```python
from build123d import *

# Parameters (mm, degrees)
SKETCH1_R           = 2.38125
SKETCH1_R_2         = 3.175
BOSS_EXTRUDE1_DEPTH = 3.175
FILLET1_R           = 7.62


with BuildPart() as part:
    # Sketch1 → Boss-Extrude1 (new body)
    with BuildSketch(Plane.XY):
        Polygon((0, 0), (25.4, 0), (25.4, -50.8), (50.8, -50.8), (50.8, -17.819677815), (65.055742252, 0), (65.055742252, 81.319677815), align=None)
        with Locations((15.875, 9.525)):
            Circle(SKETCH1_R, mode=Mode.SUBTRACT)
        with Locations((46.005742252, 38.1)):
            Circle(SKETCH1_R_2, mode=Mode.SUBTRACT)
        with Locations((46.005742252, 12.7)):
            Circle(SKETCH1_R_2, mode=Mode.SUBTRACT)
        with Locations((38.1, -12.7)):
            Circle(SKETCH1_R_2, mode=Mode.SUBTRACT)
        with Locations((38.1, -38.1)):
            Circle(SKETCH1_R_2, mode=Mode.SUBTRACT)
    extrude(amount=BOSS_EXTRUDE1_DEPTH)

    # Fillet1
    fillet1_edges = [part.edges().sort_by_distance(p)[0] for p in [
        (65.055742252, 81.319677815, 1.5875),
        (65.055742252, 0, 1.5875),
        (50.8, -17.819677815, 1.5875),
    ]]
    fillet(fillet1_edges, radius=FILLET1_R)


solid = part.part
```
Work out the finished part from the listing and answer in its coordinate system (mm). A direction names the side the tool comes from. Give positions to 0.01 mm unless a question says otherwise; leave off trailing zeros. Write each loop counter-clockwise with the first axis right and the second up, starting at its lowest first coordinate (ties: lowest second). Pieces come first, ordered by that corner, then holes.
(1) The part is cut by section D-D on y = -38.1. Write down the section's boundary in (x, z) (3 decimals), plus the area to 3 significant figures.
Final values:
outline: (25.4, 0) - (34.925, 0) - (34.925, 3.175) - (25.4, 3.175) - close; (41.275, 0) - (50.8, 0) - (50.8, 3.175) - (41.275, 3.175) - close
area: 60.5 mm2
(2) The part is cut by section B-B on x = 44. Write down the section's boundary in (y, z) (3 decimals), plus the area to 3 significant figures.
Final values:
outline: (-50.8, 0) - (10.239, 0) - (10.239, 3.175) - (-50.8, 3.175) - close; (15.161, 0) - (35.639, 0) - (35.639, 3.175) - (15.161, 3.175) - close; (40.561, 0) - (55, 0) - (55, 3.175) - (40.561, 3.175) - close
area: 305 mm2
(3) Flat-ended cylindrical pins translate along their axes: pin 1 Ø1.5 at (x, z) = (29, 1.5) entering from +Y; pin 2 Ø1.6 at (y, z) = (-23.5, 1.5) entering from -X; pin 3 Ø1 at (x, z) = (15.5, 1.5) entering from -Y. Find the tip coordinate at first contact, or state that the pin passes through.
Final values:
pin 1: stops at y = 37.19
pin 2: stops at x = 25.4
pin 3: stops at y = 0
(4) The part is cut by section C-C on z = 2. Count the separate pieces of the cut face and the enclosed holes in it, plus the area to 3 significant figures.
Final values:
separate pieces: 1
enclosed holes: 5
area: 3,820 mm2
(5) Which of the six approach directions +Z, -Z, +X, -X, +Y, -Y give full straight-line access (tool end or side, diameter ignored) to faces 1 (the flat face through (25.4, -25, 2)), 2 (the flat face through (50.8, -36, 2)), 3 (the flat face through (47, 9, 3.175))?
Final values:
face 1: +Z, -Z, -X, -Y
face 2: +Z, -Z, +X, -Y
face 3: +Z, +X, -X, +Y, -Y
(6) Straight lines are drawn through the part: line 1 (Y direction, x = 38.1, z = 0.75) (3 decimals); line 2 (Y direction, x = 40.5, z = 2.45) (3 decimals); line 3 (Y direction, x = 14, z = 1.35). For each, find the intervals that lie inside material, in ascending order.
Final values:
line 1: y = -50.8 to -41.275, -34.925 to -15.875, -9.525 to 47.625
line 2: y = -50.8 to -40.179, -36.021 to -14.779, -10.621 to 50.625
line 3: y = 0 to 8.06, 10.99 to 17.5
(7) The part is cut by section A-A on y = 38.1. Write down the section's boundary in (x, z) (3 decimals).
Final values:
outline: (30.48, 0) - (42.831, 0) - (42.831, 3.175) - (30.48, 3.175) - close; (49.181, 0) - (65.056, 0) - (65.056, 3.175) - (49.181, 3.175) - close
(8) The mould has two halves that part along X. Classify faces 4 (the cylindrical face through (18.146, 10.24, 1.565)), 5 (the flat face through (13, 0, 2)), 6 (the cylindrical face through (59.83, 66.83, 1.61)): pulls with the +X half, pulls with the -X half, needs draft (parallel to the pull), parting line crosses it, or undercut.
Final values:
face 4: undercut
face 5: needs draft
face 6: parting line crosses it
